Can you work these out from the model? Positions are in its coordinate system, mm. Round coordinates to 2 decimals unless told otherwise and drop trailing zeros. Loops run counter-clockwise (first coordinate to the right, second up) from the corner with the lowest first, then second, coordinate; pieces in that order, holes last.
(1) I want a section at C-C on z = 43. Write out the boundary of the cut face in (x, y) (1 decimal), plus the area to 3 significant figures.
(2) Will these pins go through, and if not, where does the flat tip stop? pin 1 Ø6 at (x, z) = (9.5, 263.5) entering from -Y; pin 2 Ø10 at (x, y) = (11.5, 3) entering from +Z; pin 3 Ø2 at (x, z) = (15.5, 53.5) entering from +Y; pin 4 Ø3 at (y, z) = (-16, 220.5) entering from +X.
(3) I want a section at B-B on x = -5.5. Write out the boundary of the cut face in (y, z).
(4) I want a section at A-A on y = 0. Write out the boundary of the cut face in (x, z).
(5) Thinking about a two-plate mould opening in X: for faces 1 (the face through (-4, 17, 232)), 2 (the face through (20.06, -6.32, 231.27)), 3 (the face through (-2, -18, 469.113)), which applies, released by +X, released by -X, zero draft, split by the parting line, or undercut?
(6) If I drill on line 1 along X through (y, z) = (-1.5, 285); line 2 along Y through (x, z) = (0, 121), over which ranges is the centre line in solid material (lowest first)?
Autodesk Inventor part; units mm, degrees
ref_plane "Work Plane1" through (0, 0, 0) normal (1, 0, 0) x (0, 0, 1)
ref_plane "XZ Plane" through (0, 0, 0) normal (0, 1, 0) x (-1, 0, 0)
ref_plane "XY Plane" through (0, 0, 0) normal (0, 0, 1) x (1, 0, 0)
sketch "Sketch1" plane through (0, 0, 0) normal (0, 0, 1) x (1, 0, 0)
  circle A0 centre (0, 0) radius 21.0312
  circle A1 centre (0, 0) radius 17.4625
  dimension "d0" = 34.925
  dimension "d1" = 42.0624
extrude "Extrusion1" add sketch "Sketch1" along normal blind 469.1126
ref_plane "Work Plane1" through (0, 0, 0) normal (1, 0, 0) x (0, 0, 1)
sketch "Sketch2" plane through (0, 0, 0) normal (1, 0, 0) x (0, 0, 1)
  circle A0 centre (-11.0998, 0) radius 21.4312
  line L0 (-132.8598, 0) -> (569.4413, 0)
  line L1 (469.1126, 17.4625) -> (469.1126, -17.4625)
  dimension "d5" = 42.8625
  dimension "d6" = 480.2124
extrude "Extrusion2" cut sketch "Sketch2" against normal mid plane 1066.8
sketch "Sketch3" plane through (0, 0, 0) normal (1, 0, 0) x (0, 0, 1)
  line L0 (0, -21.0312) -> (469.1126, -21.0312)
  line L1 (469.1126, 17.4625) -> (469.1126, -17.4625)
  line L2 (469.1126, 21.0312) -> (469.1126, -21.0312)
  line L3 (483.7746, -29.5638) -> (456.7933, -29.5638)
  line L4 (456.7933, -29.5638) -> (456.7933, -21.0312)
  line L5 (456.7933, -21.0312) -> (462.7626, -21.0312)
  line L6 (469.1126, -14.6812) -> (469.1126, -8.6172)
  line L7 (469.1126, -8.6172) -> (483.7746, -8.6172)
  line L8 (483.7746, -8.6172) -> (483.7746, -29.5638)
  arc A0 (462.7626, -21.0312) -> (469.1126, -14.6812) centre (462.7626, -14.6812) ccw
  dimension "d9" = 6.35
extrude "Extrusion3" cut sketch "Sketch3" against normal mid plane 1066.8
properties part number "FE-00006-10"
Filled sheet:
1. outline: circle Ø42.1 at (0, 0); hole circle Ø34.9 at (0, 0)
1. area: 432 mm2
2. pin 1: stops at y = -20
2. pin 2: passes through
2. pin 3: stops at y = 15.23
2. pin 4: stops at x = 15.23
3. outline: (-20.3, 0) - (-18.33, 0) arc R21.43 cw to (-16.57, 2.49) - (-16.57, 469.11) - (-20.3, 469.11) - close; (16.57, 2.49) arc R21.43 cw to (18.33, 0) - (20.3, 0) - (20.3, 465.72) arc R6.35 ccw to (16.57, 468.82) - close
4. outline: (-21.03, 10.33) - (-17.46, 10.33) - (-17.46, 469.11) - (-21.03, 469.11) - close; (17.46, 10.33) - (21.03, 10.33) - (21.03, 469.11) - (17.46, 469.11) - close
5. face 1: undercut
5. face 2: split by the parting line
5. face 3: zero draft
6. line 1: x = -20.98 to -17.4, 17.4 to 20.98
6. line 2: y = -21.03 to -17.46, 17.46 to 21.03
